Autodesk Inventor part; units mm, degrees
ref_plane "IDS_WORKPLANE{1}" through (-4.6, 0, 0) normal (1, 0, 0) x (0, 0, -1)
ref_plane "Work Plane2" through (69.85, 0, 0) normal (0, 0, -1) x (1, 0, 0)
ref_plane "YZ Plane" through (0, 0, 0) normal (1, 0, 0) x (0, 1, 0)
sketch "Sketch1" plane through (0, 0, 0) normal (0, 0, 1) x (1, 0, 0)
  line L0 (-0.59, 0) -> (16, 0)
  line L1 (16, 0) -> (16, 3)
  line L2 (16, 3) -> (0, 3)
  line L3 (0, 3) -> (0, 6)
  line L4 (-9.3003, 0) -> (20.2167, 0)
  line L5 (0, -1.2172) -> (0, 7.3031)
  line L6 (-4.6, 2.3998) -> (-5.0836, 2.3998) construction
  line L7 (-4.6, 0) -> (-0.59, 0)
  line L8 (0, 0) -> (-0.59, 0)
  line L9 (-4.6, 0) -> (-4.6, 6)
  arc A0 (-2.8922, 6) -> (-4.6, 2.3998) centre (5.1078, 0) ccw
  line L10 (-4.6, 6) -> (0, 6)
  dimension "d0" = 16
  dimension "d1" = 6
  dimension "d2" = 12
  dimension "d4" = 4.7996
  dimension "d13" = 4.6
  dimension "d14" = 4.01
  dimension "d46" = 10
  dimension "d47" = 0
revolve "Body" add sketch "Sketch1" angle 360 about axis through (-0.59, 0, 0) along (1, 0, 0) contours L4 L9 A0 L10 L3 L5 L0 | L5 L2 L1 L0
ref_plane "IDS_WORKPLANE{1}" through (-4.6, 0, 0) normal (1, 0, 0) x (0, 0, -1)
sketch "Sketch2" plane through (-4.6, 0, 0) normal (1, 0, 0) x (0, 0, -1)
  line L0 (0, -8.4) -> (0, 8.4)
  line L1 (8.4, 0) -> (-8.4, 0)
  line L2 (-1.289, 1.289) -> (1.289, 1.289)
  line L3 (1.289, 1.289) -> (1.289, -1.289)
  line L4 (1.289, -1.289) -> (-1.289, -1.289)
  line L5 (-1.289, -1.289) -> (-1.289, 1.289)
  line L6 (0, 1.289) -> (0, -1.289) construction
  line L7 (-1.289, 0) -> (1.289, 0) construction
  dimension "d7" = 2.578
  dimension "d9" = 2.578
extrude "Extrusion" cut sketch "Sketch2" along normal blind 4.01
fillet "Fillet1" radius 1.289 4 edges at (-0.59, 0, -1.289) (-0.59, -1.289, 0) (-0.59, 0, 1.289) (-0.59, 1.289, 0)
chamfer "Chamfer1" distance 0.401 angle 45 4 edges at (-4.6, 1.289, 0) (-4.6, 0, -1.289) (-4.6, -1.289, 0) (-4.6, 0, 1.289)
thread "Thread"
chamfer "Chamfer2" distance 0.875 distance2 0.6135 1 edges at (16, -3, 0) measured on face at (16, -1.1424, 0.935)
ref_plane "Work Plane2" through (69.85, 0, 0) normal (0, 0, -1) x (1, 0, 0)
fillet "Fillet2" radius 0.3 1 edges at (0, -3, 0)
equation "\"d0\" = NLG"
equation "\"d1\" = GD"
equation "\"d2\" = KOD"
equation "\"d4\" = 1.42 * KOM"
equation "\"d13\" = KOH"
equation "\"d14\" = STI"
equation "\"d46\" = KR"
equation "\"d7\" = KOM - 0.2 * STI"
equation "\"d9\" = KOM - 0.2 * STI"
equation "\"d48\" = STI"
equation "\"d50\" = -0.1 * STI + 0.5 * KOM"
equation "\"d51\" = 0.1 * STI"
equation "\"d18\" = GEL"
equation "\"d20\" = -0.5 * SPD + 0.5 * GD"
equation "\"d21\" = GUL"
equation "\"d44\" = R"
equation "\"GD\" = 6"
equation "\"NLG\" = 16"
equation "\"GEL\" = 15"
equation "\"KOD\" = 12"
equation "\"KOH\" = 4.6"
equation "\"SPD\" = 4.25"
equation "\"KR\" = 10"
equation "\"RR\" = 2"
equation "\"GUL\" = 0.61345 * PTC"
equation "\"KEWI\" = 0"
equation "\"SDM\" = 3.38"
equation "\"STI\" = 4.01"
equation "\"d6\" = -KOH"
equation "\"R\" = 0.3"
equation "\"KOM\" = 3.38"
equation "\"PTC\" = 1"
properties part number "ANSI B18.6.7M - M6x1 x 16, SRPHMSTIM" material "Steel, Mild"
Geometry: final body of the model. Coordinates: model frame, mm. A direction names the side the tool comes from. Coordinates: 2 decimals unless noted, no trailing zeros. Write each loop counter-clockwise with the first axis right and the second up, starting at its lowest first coordinate (ties: lowest second). Pieces come first, ordered by that corner, then holes. Notation, with made-up numbers: M -11,26 L 32,26 A10 ccw 32,33 Z; hole C 59,-37 d6. An arc over 180 degrees is marked long. Answer as CSV lines item,"result". Start each with the question number.
Q1. Mould query, pull axis Y, two halves, no side actions, for faces 1 (the flat face through (16, 0, 0)), 2 (the cylindrical face through (-1.13, 1.05, 0.02)), 3 (the cylindrical face through (-1, -6, 0)). Classes: released by +Y, released by -Y, zero draft, split by the parting line, or undercut.
Q2. Cut plane A-A on x = 11.75. Return the cut outline in (y, z), then the cut area to 3 significant figures.
Q3. Pin query (flat end, axial travel): P1, Ø1.5, axis at y = 4.5, z = 1, coming from the -X side; P2, Ø2, axis at y = -4.5, z = 2.5, coming from the -X side; P3, Ø5, axis at x = 13.5, z = 0.5, coming from the +Y side. Return the tip coordinate at first contact, or that it passes through.
Q4. Reachability of faces 4 (the flat face through (0, 3, -3)), 5 (the flat face through (-4.6, 0, -2)), 6 (the flat face through (-3, 1.289, 0)) from +Z, -Z, +X, -X, +Y, -Y: full face, straight path, thin tool, end or side. Return the list, or none.
Q5. Line query: line 1 (Z direction, x = -0.5, y = -0.25); line 2 (Z direction, x = -2, y = 0.5); line 3 (X direction, y = -2.5, z = 3.5). Output: solid intervals per line, ascending. Write a range as from..to.
Findings below:
1,face 1,"zero draft"
1,face 2,"undercut"
1,face 3,"split by the parting line"
2,outline,"C 0,0 d6"
2,area,"28.3 mm2"
3,P1,"stops at x = -4.12"
3,P2,"stops at x = -3.99"
3,P3,"stops at y = 3"
4,face 4,"+X"
4,face 5,"+Z, -Z, -X, +Y, -Y"
4,face 6,"-X"
5,line 1,"z = -5.99..5.99"
5,line 2,"z = -5.98..-1.29, 1.29..5.98"
5,line 3,"x = -3.92..0"
